```python
from build123d import *

# Parameters (mm, degrees)
ESQUISSE1_W                  = 256
ESQUISSE1_H                  = 204
BOSS_EXTRU_1_DEPTH           = 18
CONG_1_R                     = 8
ENL_V_MAT_EXTRU_2_DEPTH      = 328.835324515
ENL_V_MAT_EXTRU_2_DEPTH_BACK = 328.835324515


with BuildPart() as part:
    # Esquisse1 → Boss.-Extru.1 (new body)
    with BuildSketch(Plane.XY):
        with Locations((128, 102)):
            Rectangle(ESQUISSE1_W, ESQUISSE1_H)
    extrude(amount=BOSS_EXTRU_1_DEPTH)

    # Congé1
    cong_1_edges = [part.edges().sort_by_distance(p)[0] for p in [
        (128, 204, 18),
        (128, 204, 0),
    ]]
    fillet(cong_1_edges, radius=CONG_1_R)

    # Esquisse4 → Enlèv. mat.-Extru.2 (cut, two sides: drawn at the far end of the back side and taken through both)
    with BuildSketch(Plane(origin=(256, 0, 0), x_dir=(0, 0, -1), z_dir=(1, 0, 0)).offset(-ENL_V_MAT_EXTRU_2_DEPTH_BACK)):
        Polygon((0, 0), (-18, 0), (-18, 4.823085464), align=None)
    extrude(amount=ENL_V_MAT_EXTRU_2_DEPTH + ENL_V_MAT_EXTRU_2_DEPTH_BACK, mode=Mode.SUBTRACT)


solid = part.part
```
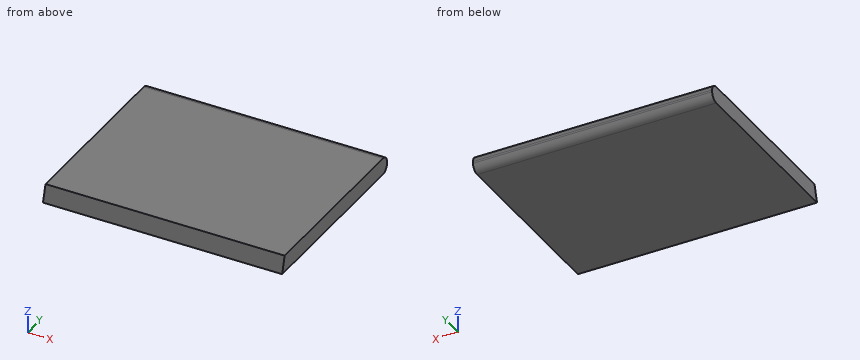
Source: CAD feature listing. Evaluate the final solid. Frame: model axes, mm. Coordinates: 2 decimals unless noted, no trailing zeros. Loops run counter-clockwise (first coordinate to the right, second up) from the corner with the lowest first, then second, coordinate; pieces in that order, holes last. Notation, with made-up numbers: M 72,21.5 L 129,21.5 A31 ccw 129,49.5 Z; hole C -15.5,13.25 d8. An arc over 180 degrees is marked long. Use a Markdown table: item, result. Add a question column.
Q1. Section query A-A, the plane x = 74.5. Return loops of the section in (y, z).
Q2. Material intervals for L1, parallel to Y at x = 113.5, z = 10.75; L2, parallel to Y at x = 201, z = 6.5, sorted ascending.
Q3. First-contact query: pin 1 (1 mm diameter, centred on y = 96.5, z = 8, fed in from -X); pin 2 (1 mm diameter, centred on x = 26.5, z = 4.5, fed in from +Y); pin 3 (1 mm diameter, centred on x = 120, z = 3.5, fed in from +Y); pin 4 (1 mm diameter, centred on x = 165.5, z = 12, fed in from -Y). Flat tips, straight axial feed; report the tip coordinate or a pass-through.
Q4. Section query B-B, the plane z = 14.25. Return loops of the section in (x, y).
Result:
| question | item | result |
|---|---|---|
| 1 | outline | M 0,0 L 196,0 A8 ccw 204,8 L 204,10 A8 ccw 196,18 L 4.82,18 Z |
| 2 | L1 | y = 2.88 to 203.96 |
| 2 | L2 | y = 1.74 to 203.86 |
| 3 | pin 1 | stops at x = 0 |
| 3 | pin 2 | stops at y = 203.42 |
| 3 | pin 3 | stops at y = 202.93 |
| 3 | pin 4 | stops at y = 3.08 |
| 4 | outline | M 0,3.82 L 256,3.82 L 256,202.78 L 0,202.78 Z |
